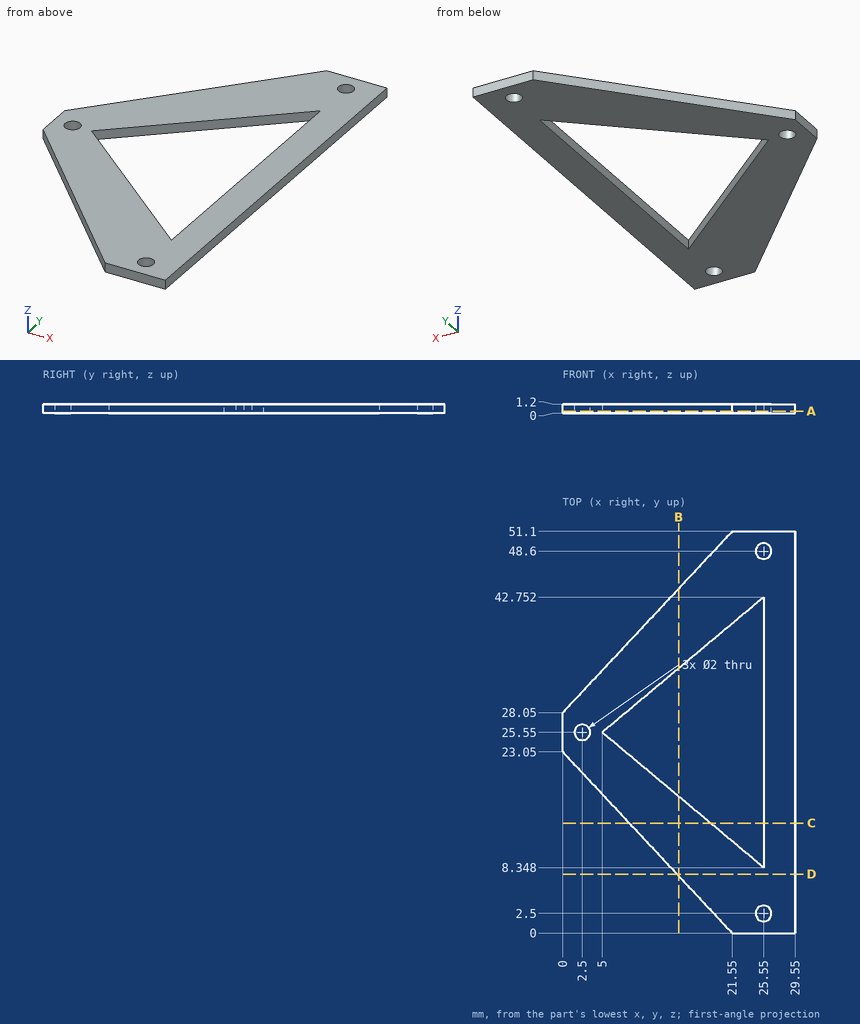
Geometry check sheet. Reference: drawing and pictorial views, mm from the part's lowest x, y, z. Give positions to 0.01 mm unless a question says otherwise; leave off trailing zeros. Order: outer loops, then holes, each group sorted by start corner. A loop starts at its lowest first (then second) coordinate and runs counter-clockwise, first axis right, second up. Notation, with made-up numbers: M 21.25,73.25 L 59.25,73.25 A25 cw 59.25,99.25 Z; hole C 53.5,37.25 d11. An arc over 180 degrees is marked long. Answer as CSV lines item,"result". Start each with the question number.
Item 1: Thickness scan on line 1 (Y direction, x = 25, z = 0.75) (1 decimal); line 2 (Y direction, x = 12, z = 0.7) (1 decimal); line 3 (Y direction, x = 20, z = 0.8) (1 decimal). Record the ranges inside material, lowest first. Write a range as [from, to].
Item 2: Cross-section at C-C on y = 14. Enter the section's corners in (x, z), plus the area to 3 significant figures.
Item 3: Cross-section at B-B on x = 14.75. Enter the section's corners in (y, z).
Item 4: Cross-section at D-D on y = 7.5. Enter the section's corners in (x, z).
Item 5: Cross-section at A-A on z = 0.3. Enter the section's corners in (x, y).
Established:
1,line 1,"y = [0, 1.7], [3.3, 8.8], [42.3, 47.8], [49.4, 51.1]"
1,line 2,"y = [10.2, 19.7], [31.4, 40.9]"
1,line 3,"y = [1.7, 13], [38.1, 49.4]"
2,outline,"M 8.46,0 L 18.8,0 L 18.8,1.2 L 8.46,1.2 Z; M 25.55,0 L 29.55,0 L 29.55,1.2 L 25.55,1.2 Z"
2,area,"17.2 mm^2"
3,outline,"M 7.27,0 L 17.39,0 L 17.39,1.2 L 7.27,1.2 Z; M 33.71,0 L 43.83,0 L 43.83,1.2 L 33.71,1.2 Z"
4,outline,"M 14.54,0 L 29.55,0 L 29.55,1.2 L 14.54,1.2 Z"
5,outline,"M 0,23.05 L 21.55,0 L 29.55,0 L 29.55,51.1 L 21.55,51.1 L 0,28.05 Z; hole C 2.5,25.55 d2; hole M 5,25.55 L 25.55,8.35 L 25.55,42.75 Z; hole C 25.55,2.5 d2; hole C 25.55,48.6 d2"
